Geometry check sheet. Reference: the model listing, model coordinates, mm. Face numbers are marked on the shaded views. A direction names the side the tool comes from. Round coordinates to 2 decimals unless told otherwise and drop trailing zeros. Write each loop counter-clockwise with the first axis right and the second up, starting at its lowest first coordinate (ties: lowest second). Pieces come first, ordered by that corner, then holes. Notation, with made-up numbers: M 50,-38.75 L 98,-38.75 A13 ccw 98,-23.75 Z; hole C 30.5,83 d1. An arc over 180 degrees is marked long. Answer in a Markdown table with one row per item. Add a question column.
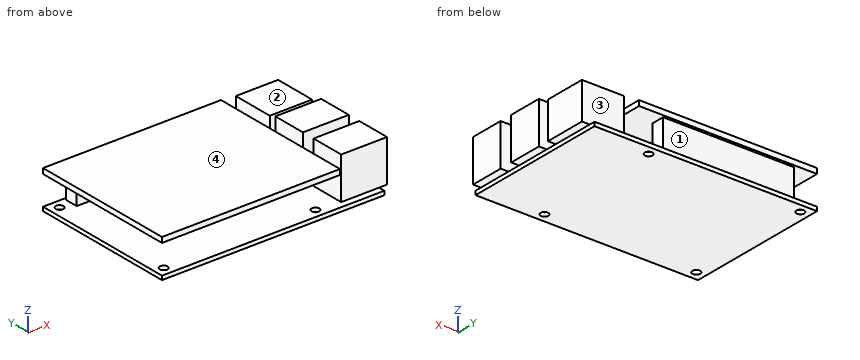
from build123d import *

# Parameters (mm, degrees)
SKETCH1_W           = 85
SKETCH1_H           = 56
BOSS_EXTRUDE1_DEPTH = 1.5
SKETCH2_R           = 1.5
CUT_EXTRUDE1_DEPTH  = 102.800049116
SKETCH3_W           = 17.5
SKETCH3_H           = 13
BOSS_EXTRUDE3_DEPTH = 16
SKETCH4_W           = 16.168614458
SKETCH4_H           = 16
BOSS_EXTRUDE4_DEPTH = 14
SKETCH5_W           = 50
SKETCH5_H           = 5
BOSS_EXTRUDE5_DEPTH = 11
SKETCH6_W           = 68
SKETCH6_H           = 56
BOSS_EXTRUDE6_DEPTH = 2


with BuildPart() as part:
    # Sketch1 → Boss-Extrude1 (new body)
    with BuildSketch(Plane.XY):
        with Locations((42.5, 28)):
            Rectangle(SKETCH1_W, SKETCH1_H)
    extrude(amount=BOSS_EXTRUDE1_DEPTH)

    # Sketch2 → Cut-Extrude1 (cut, through all)
    with BuildSketch(Plane.XY.offset(1.5)):
        with Locations((3.5, 52.5)):
            Circle(SKETCH2_R)
        with Locations((3.5, 3.5)):
            Circle(SKETCH2_R)
        with Locations((61.5, 52.5)):
            Circle(SKETCH2_R)
        with Locations((61.5, 3.5)):
            Circle(SKETCH2_R)
    extrude(amount=-CUT_EXTRUDE1_DEPTH, mode=Mode.SUBTRACT)

    # Sketch3 → Boss-Extrude3 (add)
    with BuildSketch(Plane.XY.offset(1.5)):
        with Locations((79.25, 9)):
            Rectangle(SKETCH3_W, SKETCH3_H)
        with Locations((79.25, 27)):
            Rectangle(SKETCH3_W, SKETCH3_H)
    extrude(amount=BOSS_EXTRUDE3_DEPTH)

    # Sketch4 → Boss-Extrude4 (add)
    with BuildSketch(Plane.XY.offset(1.5)):
        with Locations((79.915692771, 45.75)):
            Rectangle(SKETCH4_W, SKETCH4_H)
    extrude(amount=BOSS_EXTRUDE4_DEPTH)

    # Sketch5 → Boss-Extrude5 (add)
    with BuildSketch(Plane.XY.offset(1.5)):
        with Locations((33, 52.5)):
            Rectangle(SKETCH5_W, SKETCH5_H)
    extrude(amount=BOSS_EXTRUDE5_DEPTH)

    # Sketch6 → Boss-Extrude6 (add)
    with BuildSketch(Plane.XY.offset(12.5)):
        with Locations((34, 28)):
            Rectangle(SKETCH6_W, SKETCH6_H)
    extrude(amount=BOSS_EXTRUDE6_DEPTH)


solid = part.part
Item 1: Gauge pin test, flat ends, axial feed: pin 1 Ø1.5 at (x, y) = (86, 25.5) entering from -Z; pin 2 Ø1.5 at (x, z) = (35.5, 2.5) entering from -Y; pin 3 Ø6.5 at (y, z) = (9.5, 9) entering from -X. Record the tip position at first contact, or that the pin passes through.
Item 2: Section check C-C, the plane y = 24.5. Record the boundary of the cut face in (x, z).
Item 3: Section check A-A, the plane x = 61.5. Record the boundary of the cut face in (y, z).
Item 4: Section check B-B, the plane y = 52.5. Record the boundary of the cut face in (x, z), and give its area (3 significant figures).
Item 5: Access from +Z, -Z, +X, -X, +Y, -Y to the whole of each face (thin tool, end or side, straight path). Record for the marked faces 1, 2, 3 and 4.
Item 6: Section check D-D, the plane z = 8. Record the boundary of the cut face in (x, y), and give its area (3 significant figures).
Item 7: Scan lines: probe 1 along Y at (x, z) = (61.5, 0.5); probe 2 along Z at (x, y) = (64.5, 44.5); probe 3 along X at (y, z) = (47, 2.5). Record each from-to range of solid material in increasing order. Write a range as from..to.
Result sheet:
| question | item | result |
|---|---|---|
| 1 | pin 1 | stops at z = 1.5 |
| 1 | pin 2 | stops at y = 50 |
| 1 | pin 3 | stops at x = 70.5 |
| 2 | outline | M 0,0 L 85,0 L 85,1.5 L 88,1.5 L 88,17.5 L 70.5,17.5 L 70.5,1.5 L 0,1.5 Z; M 0,12.5 L 68,12.5 L 68,14.5 L 0,14.5 Z |
| 3 | outline | M 0,0 L 2,0 L 2,1.5 L 0,1.5 Z; M 0,12.5 L 56,12.5 L 56,14.5 L 0,14.5 Z; M 5,0 L 51,0 L 51,1.5 L 5,1.5 Z; M 54,0 L 56,0 L 56,1.5 L 54,1.5 Z |
| 4 | outline | M 0,0 L 2,0 L 2,1.5 L 0,1.5 Z; M 0,12.5 L 8,12.5 L 8,1.5 L 5,1.5 L 5,0 L 60,0 L 60,1.5 L 58,1.5 L 58,12.5 L 68,12.5 L 68,14.5 L 0,14.5 Z; M 63,0 L 85,0 L 85,1.5 L 88,1.5 L 88,15.5 L 71.83,15.5 L 71.83,1.5 L 63,1.5 Z |
| 4 | area | 1,030 mm^2 |
| 5 | face 1 | +X, -X, +Y |
| 5 | face 2 | +Z, +X, -X, +Y |
| 5 | face 3 | +Z, +X, +Y |
| 5 | face 4 | +Z, -X, +Y, -Y |
| 6 | outline | M 8,50 L 58,50 L 58,55 L 8,55 Z; M 70.5,2.5 L 88,2.5 L 88,15.5 L 70.5,15.5 Z; M 70.5,20.5 L 88,20.5 L 88,33.5 L 70.5,33.5 Z; M 71.83,37.75 L 88,37.75 L 88,53.75 L 71.83,53.75 Z |
| 6 | area | 964 mm^2 |
| 7 | probe 1 | y = 0..2, 5..51, 54..56 |
| 7 | probe 2 | z = 0..1.5, 12.5..14.5 |
| 7 | probe 3 | x = 71.83..88 |
